```python
from build123d import *

# Parameters (mm, degrees)
F2_R     = 9.525
F3_DEPTH = 19.05


with BuildPart() as f1:
    # F0 (on Front) → F1 (revolve)
    with BuildSketch(Plane.XZ):
        Polygon((-76.2, 0), (-6.35, 0), (-6.35, 38.1), (-12.7, 38.1), (-12.7, 50.8), (-25.4, 50.8), (-25.4, 19.05), (-63.5, 19.05), (-63.5, 76.2), (-76.2, 76.2), align=None)
    revolve(axis=Axis((0, 0, 38.1), (0, 0, 1)))

    # F2 (on Top) → F3 (join)
    with BuildSketch(Plane.XY):
        with BuildLine():
            Line((-107.95, -76.2), (0, -76.2))
            ThreePointArc((0, -76.2), (-53.8815367264, -53.8815367264), (-76.2, 0))
            Line((-76.2, 0), (-76.2, -38.1))
            Line((-76.2, -38.1), (-107.95, -38.1))
            Line((-107.95, -38.1), (-107.95, -47.625))
            ThreePointArc((-107.95, -47.625), (-101.2148079092, -50.4148079092), (-98.425, -57.15))
            ThreePointArc((-98.425, -57.15), (-101.2148079092, -63.8851920908), (-107.95, -66.675))
            Line((-107.95, -66.675), (-107.95, -76.2))
        make_face()
        with BuildLine():
            ThreePointArc((-107.95, -38.1), (-127, -57.15), (-107.95, -76.2))
            Line((-107.95, -76.2), (-107.95, -66.675))
            ThreePointArc((-107.95, -66.675), (-117.475, -57.15), (-107.95, -47.625))
            Line((-107.95, -47.625), (-107.95, -38.1))
        make_face()
        with BuildLine():
            Line((-76.2, 38.1), (-76.2, 0))
            ThreePointArc((-76.2, 0), (-53.8815367264, 53.8815367264), (0, 76.2))
            Line((0, 76.2), (-107.95, 76.2))
            ThreePointArc((-107.95, 76.2), (-127, 57.15), (-107.95, 38.1))
            Line((-107.95, 38.1), (-76.2, 38.1))
        make_face()
        with Locations((-107.95, 57.15)):
            Circle(F2_R, mode=Mode.SUBTRACT)
        with BuildLine():
            ThreePointArc((0, 76.2), (53.8815367264, 53.8815367264), (76.2, 0))
            Line((76.2, 0), (76.2, 38.1))
            Line((76.2, 38.1), (107.95, 38.1))
            ThreePointArc((107.95, 38.1), (127, 57.15), (107.95, 76.2))
            Line((107.95, 76.2), (0, 76.2))
        make_face()
        with Locations((107.95, 57.15)):
            Circle(F2_R, mode=Mode.SUBTRACT)
        with BuildLine():
            ThreePointArc((76.2, 0), (53.8815367264, -53.8815367264), (0, -76.2))
            Line((0, -76.2), (107.95, -76.2))
            ThreePointArc((107.95, -76.2), (127, -57.15), (107.95, -38.1))
            Line((107.95, -38.1), (76.2, -38.1))
            Line((76.2, -38.1), (76.2, 0))
        make_face()
        with Locations((107.95, -57.15)):
            Circle(F2_R, mode=Mode.SUBTRACT)
    extrude(amount=F3_DEPTH)


solid = f1.part
```
Can you work these out from the model? Positions are in its coordinate system, mm. A direction names the side the tool comes from. Give positions to 0.01 mm unless a question says otherwise; leave off trailing zeros. Order: outer loops, then holes, each group sorted by start corner. A loop starts at its lowest first (then second) coordinate and runs counter-clockwise, first axis right, second up. Notation, with made-up numbers: M 81.25,11.25 L 121.25,11.25 A23 cw 121.25,37.25 Z; hole C 44,38.5 d6. An arc over 180 degrees is marked long. Write item = value, one per line. Start each with the question number.
Q1. Suppose I cut it at B-B (y = 57.15). Write out the boundary of the cut face in (x, z) (3 decimals).
Q2. We'd pull the mould along X, two halves only. Please class faces 5 (the cylindrical face through (112.35, 48.7, 9.39)), 6 (the cylindrical face through (60.47, 46.367, 47.225)), 7 (the flat face through (82, -60, 19.05)): pulls with the +X half, pulls with the -X half, needs draft (parallel to the pull), parting line crosses it, or undercut.
Q3. Suppose I cut it at A-A (z = 11.5). Write out the boundary of the cut face in (x, y) (3 decimals).
Q4. I need wall thicknesses on probe 1 along X at (y, z) = (0, 45); probe 2 along Y at (x, z) = (-107.95, 10.25) (3 decimals); probe 3 along Y at (x, z) = (107, 7). Which ranges of each line are inside material? Lowest first, please. Write a range as [from, to].
Q5. Suppose I cut it at C-C (z = 27). Write out the boundary of the cut face in (x, y).
Q6. Suppose I cut it at D-D (x = -28). Write out the boundary of the cut face in (y, z), plus the area to 3 significant figures.
Q7. Will these pins go through, and if not, where does the flat tip stop? pin 1 Ø4 at (x, y) = (54, -27) entering from +Z; pin 2 Ø11.5 at (x, y) = (-107.95, -57.15) entering from +Z; pin 3 Ø21 at (y, z) = (5.5, 9) entering from -X; pin 4 Ø1.5 at (y, z) = (-9, 24) entering from +X.
Q8. For faces 1 (the flat face through (5, -12, 50.8)), 2 (the flat face through (92, -38.1, 9)), 3 (the flat face through (82, 61, 19.05)), 4 (the flat face through (-92, 38.1, 9)), which set-ups out of +Z, -Z, +X, -X, +Y, -Y let a thin tool reach every point of the face, with its end or its side?
Check result:
q1.outline = M -127,0 L -117.475,0 L -117.475,19.05 L -127,19.05 Z; M -98.425,0 L 98.425,0 L 98.425,19.05 L 50.402,19.05 L 50.402,76.2 L 27.679,76.2 L 27.679,19.05 L -27.679,19.05 L -27.679,76.2 L -50.402,76.2 L -50.402,19.05 L -98.425,19.05 Z; M 117.475,0 L 127,0 L 127,19.05 L 117.475,19.05 Z
q2.face_5 = undercut
q2.face_6 = parting line crosses it
q2.face_7 = needs draft
q3.outline = M -107.95,-76.2 L 107.95,-76.2 A19.05 ccw 107.95,-38.1 L 76.2,-38.1 L 76.2,38.1 L 107.95,38.1 A19.05 ccw 107.95,76.2 L -107.95,76.2 A19.05 ccw -107.95,38.1 L -76.2,38.1 L -76.2,-38.1 L -107.95,-38.1 A19.05 ccw Z; hole C -107.95,-57.15 d19.05; hole C -107.95,57.15 d19.05; hole C 0,0 d12.7; hole C 107.95,-57.15 d19.05; hole C 107.95,57.15 d19.05
q4.probe_1 = [-76.2, -63.5], [-25.4, -12.7], [12.7, 25.4], [63.5, 76.2]
q4.probe_2 = [-76.2, -66.675], [-47.625, -38.1], [38.1, 47.625], [66.675, 76.2]
q4.probe_3 = [-76.2, -66.63], [-47.67, -38.1], [38.1, 47.67], [66.63, 76.2]
q5.outline = C 0,0 d152.4; C 0,0 d50.8; hole C 0,0 d127; hole C 0,0 d12.7
q6.outline = M -76.2,0 L 76.2,0 L 76.2,19.05 L 70.87,19.05 L 70.87,76.2 L 56.99,76.2 L 56.99,19.05 L -56.99,19.05 L -56.99,76.2 L -70.87,76.2 L -70.87,19.05 L -76.2,19.05 Z
q6.area = 4,490 mm2
q7.pin_1 = 19.05
q7.pin_2 = through
q7.pin_3 = -76.2
q7.pin_4 = 75.75
q8.face_1 = +Z
q8.face_2 = +Z, -Z, +X
q8.face_3 = +Z, +X, +Y
q8.face_4 = +Z, -Z, -X
